Autodesk Inventor part; units mm, degrees
ref_plane "YZ Plane" through (0, 0, 0) normal (1, 0, 0) x (0, 1, 0)
ref_plane "XZ Plane" through (0, 0, 0) normal (0, 1, 0) x (-1, 0, 0)
ref_plane "XY Plane" through (0, 0, 0) normal (0, 0, 1) x (1, 0, 0)
sketch "Sketch1" plane through (0, 0, 0) normal (0, 1, 0) x (-1, 0, 0)
  line L0 (0, 0) -> (76.2, 0)
  line L1 (76.2, 0) -> (76.2, -76.2)
  line L2 (76.2, -76.2) -> (0, -76.2)
  line L3 (0, -76.2) -> (0, 0)
  dimension "d0" = 76.2
  dimension "d1" = 76.2
extrude "Extrusion1" add sketch "Sketch1" along normal blind 50.8
sketch "Sketch2" plane through (0, 50.8, 0) normal (0, 1, 0) x (1, 0, 0)
  line L0 (0, 76.2) -> (-76.2, 76.2)
  line L1 (-76.2, 76.2) -> (-76.2, 0)
  line L2 (-76.2, 0) -> (0, 0)
  line L3 (0, 0) -> (0, 76.2)
  line L4 (-73.025, 73.025) -> (-3.175, 73.025)
  line L5 (-3.175, 73.025) -> (-3.175, 3.175)
  line L6 (-3.175, 3.175) -> (-73.025, 3.175)
  line L7 (-73.025, 3.175) -> (-73.025, 73.025)
  dimension "d4" = 3.175
  dimension "d5" = 3.175
  dimension "d6" = 3.175
  dimension "d7" = 3.175
extrude "Extrusion2" cut sketch "Sketch2" against normal blind 47.625 contours L4 L5 L6 L7
sketch "Sketch3" plane through (0, 0, 0) normal (1, 0, 0) x (0, 0, -1)
  line L0 (0, 0) -> (76.2, 0)
  line L1 (76.2, 0) -> (76.2, 50.8)
  line L2 (0, 50.8) -> (76.2, 50.8)
  line L3 (0, 0) -> (0, 50.8)
  circle A0 centre (38.1, 25.4) radius 6.35
  dimension "d10" = 12.7
extrude "Extrusion3" cut sketch "Sketch3" against normal through all contours A0
properties part number "FakeHousing"
Here's how the part is built. I have some questions about the finished solid (model axes, mm). A direction names the side the tool comes from. Give positions to 0.01 mm unless a question says otherwise; leave off trailing zeros. Order: outer loops, then holes, each group sorted by start corner. A loop starts at its lowest first (then second) coordinate and runs counter-clockwise, first axis right, second up. Notation, with made-up numbers: (34, 72) - (53, 72) arc R28 ccw to (53, 110) - close; hole circle Ø10 at (35.25, 14.5). An arc over 180 degrees is marked (long way). Answer as a JSON object with one key per item and string values. Group by question number.
Item 1: If we section it at D-D on x = -33: Please give me the cut outline in (y, z) (3 decimals), and give its area (3 significant figures).
Item 2: Which directions (+Z, -Z, +X, -X, +Y, -Y) give clear straight access to the entire face, cutting with the end or side of a thin tool? Please do faces 5 (the cylindrical face through (-74.59, 25.679, -31.756)), 6 (the flat face through (-39, 27, -73.025)).
Item 3: If we section it at B-B on y = 25.4: Please give me the cut outline in (x, z) (3 decimals).
Item 4: For P1, Ø21, axis at x = -44, z = -53.5, coming from the +Y side (3 decimals), with a flat end and sliding along its axis, tell me the tip position at first contact or that it passes through.
Item 5: If we mould it in two halves opening along Z, with no side actions, what happens to faces 1 (the flat face through (-39, 25, -76.2)), 2 (the flat face through (-76.2, 25, -46)), 3 (the flat face through (-38, 25, 0)), 4 (the cylindrical face through (-1.565, 25.679, -31.756))? For each: pulls with the +Z half, pulls with the -Z half, needs draft (parallel to the pull), parting line crosses it, or undercut.
Item 6: Please list where these lines run through material, in increasing order: probe 1 along Y at (x, z) = (-2, -38); probe 2 along X at (y, z) = (33, -13) (3 decimals).
Item 7: If we section it at C-C on y = 10: Please give me the cut outline in (x, z) (3 decimals).
Item 8: If we section it at A-A on z = -38.1: Please give me the cut outline in (x, y) (3 decimals).
Result set:
{
 "1": {"outline": "(0, -76.2) - (50.8, -76.2) - (50.8, -73.025) - (3.175, -73.025) - (3.175, -3.175) - (50.8, -3.175) - (50.8, 0) - (0, 0) - close", "area": "544 mm²"},
 "2": {"face 5": "+X, -X", "face 6": "+Y"},
 "3": {"outline": "(-76.2, -76.2) - (0, -76.2) - (0, -44.45) - (-3.175, -44.45) - (-3.175, -73.025) - (-73.025, -73.025) - (-73.025, -44.45) - (-76.2, -44.45) - close; (-76.2, -31.75) - (-73.025, -31.75) - (-73.025, -3.175) - (-3.175, -3.175) - (-3.175, -31.75) - (0, -31.75) - (0, 0) - (-76.2, 0) - close"},
 "4": {"P1": "y = 3.175"},
 "5": {"face 1": "pulls with the -Z half", "face 2": "needs draft", "face 3": "pulls with the +Z half", "face 4": "undercut"},
 "6": {"probe 1": "0 to 19.05, 31.75 to 50.8", "probe 2": "-76.2 to -73.025, -3.175 to 0"},
 "7": {"outline": "(-76.2, -76.2) - (0, -76.2) - (0, 0) - (-76.2, 0) - close; hole (-73.025, -73.025) - (-3.175, -73.025) - (-3.175, -3.175) - (-73.025, -3.175) - close"},
 "8": {"outline": "(-76.2, 0) - (0, 0) - (0, 19.05) - (-3.175, 19.05) - (-3.175, 3.175) - (-73.025, 3.175) - (-73.025, 19.05) - (-76.2, 19.05) - close; (-76.2, 31.75) - (-73.025, 31.75) - (-73.025, 50.8) - (-76.2, 50.8) - close; (-3.175, 31.75) - (0, 31.75) - (0, 50.8) - (-3.175, 50.8) - close"}
}
